Autodesk Fusion 360 part; units mm, degrees
sketch "Sketch1" plane through (0, 0, 0) normal (0, 1, 0) x (1, 0, 0)
  line L0 (-10, 10) -> (10, 10)
  line L1 (10, 10) -> (10, -10)
  line L2 (10, -10) -> (-10, -10)
  line L3 (-10, -10) -> (-10, 10)
  line L4 (-10, 10) -> (10, -10) construction
  line L5 (10, 10) -> (-10, -10) construction
  line L6 (20, 20) -> (20, -20)
  line L7 (20, -20) -> (-20, -20)
  line L8 (-20, -20) -> (-20, 20)
  line L9 (-20, 20) -> (20, 20)
  dimension "d1" = 20
  dimension "d2" = 20
  dimension "d3" = -10
extrude "Extrude1" add sketch "Sketch1" along normal blind 50 makes body 1
sketch "Sketch2" plane through (0, 50, 0) normal (0, 1, 0) x (-1, 0, 0)
  line L0 (-10, 10) -> (10, 10)
  line L1 (10, 10) -> (10, -10)
  line L2 (10, -10) -> (-10, -10)
  line L3 (-10, -10) -> (-10, 10)
  line L4 (20, -20) -> (20, 20)
  line L5 (20, 20) -> (-20, 20)
  line L6 (-20, 20) -> (-20, -20)
  line L7 (-20, -20) -> (20, -20)
ref_plane "WorkPlane1" through (-10, 25, -10) normal (-0.7071, 0, 0.7071) x (0, 1, 0)
ref_plane "WorkPlane2" through (-15.3033, 25, -4.6967) normal (-0.7071, 0, 0.7071) x (0, 1, 0)
split "Split1" by plane through (-15.3033, 25, -4.6967) normal (-0.7071, 0, 0.7071) bodies 1 makes body 2 at (-0.4044, 16.6667, 20)
ref_plane "WorkPlane3" through (20, 25, -20) normal (-0.7071, 0, 0.7071) x (0, 1, 0)
sketch "Sketch3" plane through (20, 25, -20) normal (-0.7071, 0, 0.7071) x (0, 1, 0)
  line L0 (25, -10) -> (-25, -10)
  line L1 (-25, -10) -> (-25, 10)
  line L2 (-25, 10) -> (25, 10)
  line L3 (25, 10) -> (25, -10)
extrude "Extrude2" add sketch "Sketch3" along normal blind 13 and the other way blind 0 bodies 1
sketch "Sketch4" plane through (20, 0, -20) normal (0.7071, 0, -0.7071) x (-0.7071, 0, -0.7071)
  line L0 (-10, 0) -> (10, 0)
  line L1 (10, 0) -> (10, 50)
  line L2 (10, 50) -> (-10, 50)
  line L3 (-10, 50) -> (-10, 0)
  circle A0 centre (0, 25) radius 3.14
  dimension "d13" = 6.28
ref_plane "WorkPlane4" through (12.9289, 25, -12.9289) normal (0.7071, 0, -0.7071) x (-0.7071, 0, -0.7071)
sketch "Sketch5" plane through (12.9289, 25, -12.9289) normal (0.7071, 0, -0.7071) x (-0.7071, 0, -0.7071)
  circle A0 centre (0, 0) radius 1.57
  dimension "d15" = 3.14
loft "Loft1" cut profiles "Sketch4", "Sketch5" section 1 contours A0 section 2 bodies 1
sketch "Sketch6" plane through (0, 0, -20) normal (0, 0, -1) x (-1, 0, 0)
  line L0 (-5.8579, 50) -> (-5.8579, 0)
  line L1 (-5.8579, 0) -> (20, 0)
  line L2 (20, 0) -> (20, 50)
  line L3 (20, 50) -> (-5.8579, 50)
  line L4 (10, 0) -> (-10, 0)
  line L5 (-10, 0) -> (-10, 50)
  line L6 (-10, 50) -> (10, 50)
  line L7 (10, 50) -> (10, 0)
  line L8 (10, 25) -> (-10, 25) construction
  line L9 (10, 12.5) -> (-10, 12.5) construction
  line L10 (0, 0) -> (0, 25) construction
  circle A0 centre (0, 12.5) radius 2.5
  circle A1 centre (0, 37.5) radius 2.5
  dimension "d16" = 5
extrude "Extrude3" cut sketch "Sketch6" against normal blind 21 contours A0 | A1 bodies 1
sketch "Sketch7" plane through (0, 0, 0) normal (0, -1, 0) x (1, 0, 0)
  line L0 (12.9289, -27.0711) -> (27.0711, -12.9289)
  line L1 (27.0711, -12.9289) -> (20, -5.8579)
  line L2 (20, -5.8579) -> (20, 20)
  line L3 (20, 20) -> (9.3934, 20)
  line L4 (9.3934, 20) -> (-0.6066, 10)
  line L5 (-0.6066, 10) -> (10, 10)
  line L6 (10, 10) -> (10, -10)
  line L7 (10, -10) -> (-10, -10)
  line L8 (-10, -10) -> (-10, 0.6066)
  line L9 (-10, 0.6066) -> (-20, -9.3934)
  line L10 (-20, -9.3934) -> (-20, -20)
  line L11 (-20, -20) -> (5.8579, -20)
  line L12 (5.8579, -20) -> (12.9289, -27.0711)
  circle A0 centre (-10, -10) radius 1
  circle A1 centre (10, 10) radius 1
  dimension "d21" = 2
  dimension "d22" = 2
extrude "Extrude4" cut sketch "Sketch7" against normal blind 53 contours L7 L8 A0 | L5 L6 A1 picked at (-9.3369, -10.0489) picked at (10, 10.6648) bodies 1
chamfer "Chamfer1" distance 3 angle 45 16 edges at (20, 25, 20) (27.0711, 25, -12.9289) (12.9289, 25, -27.0711) (20, 50, -20) (20, 0, -20) (20, 50, 7.0711) (23.5355, 50, -9.3934) (9.3934, 50, -23.5355) (-7.0711, 50, -20) (-20, 25, -20) (-7.0711, 0, -20) (9.3934, 0, -23.5355) (-20, 0, -14.6967) (14.6967, 0, 20) (-20, 50, -14.6967) (14.6967, 50, 20) on bodies 1
chamfer "Chamfer2" distance 2 angle 45 2 edges at (20, 0, 5.5711) (22.4749, 0, -8.3327) on bodies 1
extrude "Extrude5" cut 1 faces at (13.1588, 25.9211, -12.6991) along direction (-0.707107, 0, 0.707107) blind 17 on bodies 1 bodies 1
hidden bodies 2
equation "d1 = sqUARELENGTH"
equation "d2 = sqUARELENGTH"
equation "d3 = shellthickness"
equation "shellthickness = -10 mm"
equation "sqUARELENGTH = 20 mm"
The model under review builds one solid part; all positions refer to its coordinate system, in mm. A direction names the side the tool comes from. Round coordinates to 2 decimals unless told otherwise and drop trailing zeros. Loops run counter-clockwise (first coordinate to the right, second up) from the corner with the lowest first, then second, coordinate; pieces in that order, holes last. Notation, with made-up numbers: M -11,10.5 L 5,10.5 A29 cw 5,38.5 Z; hole C 29,43.25 d5. An arc over 180 degrees is marked long. Answer as a JSON object with one key per item and string values.
Item 1: Clearance check with flat-ended pins moving along their axes: P1, Ø5.5, axis at y = 25.5, z = 3, coming from the -X side; P2, Ø5, axis at x = 4, y = 16.5, coming from the -Z side; P3, Ø18.5, axis at y = 31.5, z = 3, coming from the +X side; P4, Ø1.8, axis at x = -10, z = -10, coming from the +Y side. State where each tip first meets the part, or that it passes through.
Check sheet entries:
{"P1": "x = -10.36", "P2": "z = -20.64", "P3": "x = 20.39", "P4": "through"}
Item 2: Tool access review of faces 5 (the face through (0.54, 35.06, -15.07)), 6 (the face through (0, 25, -10)), 7 (the face through (-10, 25, -4)): name each direction out of +Z, -Z, +X, -X, +Y, -Y from which nothing blocks a thin tool from reaching the whole face with its end or side.
Check sheet entries:
{"face 5": "-Z", "face 6": "+Y, -Y", "face 7": "+Z, +Y, -Y"}
Item 3: We need section B-B, the plane x = 1. State the section outline as (y, z) points.
Check sheet entries:
{"outline": "M 0,-17 L 3,-20 L 10.21,-20 L 10.21,-10 L 0,-10 Z; M 0,10 L 50,10 L 50,11.61 L 0,11.61 Z; M 14.79,-20 L 35.21,-20 L 35.21,-10 L 14.79,-10 Z; M 39.79,-20 L 47,-20 L 50,-17 L 50,-10 L 39.79,-10 Z"}
Item 4: We need section A-A, the plane y = 37.5. State the section outline as (x, z) points, and give its area (3 significant figures).
Check sheet entries:
{"outline": "M -20,-17 L -17,-20 L -2.5,-20 L -2.5,-10 L -9,-10 A1 cw long -10,-9 L -10,0.61 L -20,-9.39 Z; M -0.61,10 L 9,10 A1 cw long 10,9 L 10,-10 L 2.5,-10 L 2.5,-20 L 5.86,-20 L 10.81,-24.95 L 15.05,-24.95 L 24.95,-15.05 L 24.95,-10.81 L 20,-5.86 L 20,17 L 17,20 L 9.39,20 Z", "area": "839 mm2"}
Item 5: The part is to be moulded in two halves that separate along X. For faces 1 (the face through (19.71, 1.48, -18.14)), 2 (the face through (4, 25, 10)), 3 (the face through (10.4, 23.6, -11.4)), 4 (the face through (-18, 2, -18)), say which applies: +X half, -X half, draft (parallel to the pull), parting line (faces both ways), or undercut.
Check sheet entries:
{"face 1": "+X half", "face 2": "draft", "face 3": "undercut", "face 4": "-X half"}
Item 6: For line 1 along Y through (x, z) = (0, -16); line 2 along Z through (x, y) = (-7, 14); line 3 along Z through (x, y) = (6.5, 46), list the stretches that pass through material, from the lowest coordinate up.
Check sheet entries:
{"line 1": "0 to 10, 15 to 35, 40 to 50", "line 2": "-20 to -10", "line 3": "-20.64 to -10, 10 to 17.11"}
Item 7: We need section D-D, the plane z = -18. State how many separate pieces and enclosed holes the cut face has, and give its area (3 significant figures).
Check sheet entries:
{"separate pieces": "1", "enclosed holes": "2", "area": "1,910 mm2"}
Item 8: We need section C-C, the plane z = 7.5. State the section outline as (x, y) points.
Check sheet entries:
{"outline": "M 10,0 L 18,0 L 20,2 L 20,47 L 17,50 L 10,50 Z"}
